For this review, take the finished solid that the model builds, in its own axes (mm). Face numbers are marked on the shaded views. A direction names the side the tool comes from. Round coordinates to 2 decimals unless told otherwise and drop trailing zeros. Loops run counter-clockwise (first coordinate to the right, second up) from the corner with the lowest first, then second, coordinate; pieces in that order, holes last. Notation, with made-up numbers: M 29.25,-28 L 83.25,-28 A14 cw 83.25,-13 Z; hole C 7,-20 d1. An arc over 180 degrees is marked long. One line per question, with ' | ' between items. Start each with the question number.
1) For pin 1 Ø1 at (y, z) = (1, 0) entering from -X; pin 2 Ø1.5 at (y, z) = (1, -8) entering from -X; pin 3 Ø1.5 at (x, y) = (-2, -2) entering from -Z, all flat-tipped, find the tip position at first contact; note any pin that passes through.
2) For the marked faces 1 and 2, list the 3-axis set-ups (+Z, -Z, +X, -X, +Y, -Y) from which the entire face can be reached by the end or side of a thin tool; tool diameter is ignored.
3) We need section A-A (y = 0). Give the boundary of the cut face in (x, z), and give its area (3 significant figures).
4) We need section B-B (z = 7.75). Give the boundary of the cut face in (x, y), and give its area (3 significant figures).
5) For probe 1 along X at (y, z) = (-0.1, 3.25); probe 2 along Z at (x, y) = (-0.9, 0.1); probe 3 along Z at (x, y) = (-2.15, 1.65), list the stretches that pass through material, from the lowest coordinate up. Write a range as from..to.
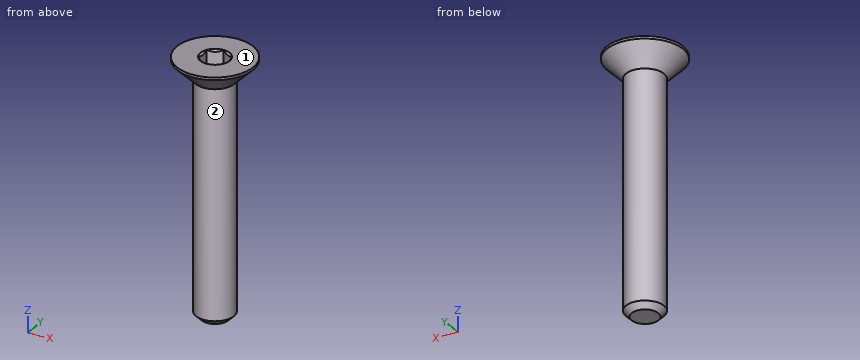
```python
from build123d import *

# Parameters (mm, degrees)
SKETCH3_W          = 20
SKETCH3_H          = 1.5
CHAMFER1_SIZE      = 0.45
CUT_EXTRUDE1_DEPTH = 1.19


with BuildPart() as part:
    # Sketch3 → Revolve1 (revolve)
    with BuildSketch(Plane(origin=(0, 0, 0), x_dir=(0, 0, -1), z_dir=(1, 0, 0))):
        with Locations((0, 0.75)):
            Rectangle(SKETCH3_W, SKETCH3_H)
    revolve(axis=Axis((0, 0, -10), (0, 0, 1)))

    # Chamfer1
    chamfer1_edges = [part.edges().sort_by_distance(p)[0] for p in [
        (0, -1.5, -10),
    ]]
    chamfer(chamfer1_edges, length=CHAMFER1_SIZE)

    # Sketch6 → Revolve2 (revolve)
    with BuildSketch(Plane(origin=(0, 0, 0), x_dir=(0, 0, -1), z_dir=(1, 0, 0))):
        Polygon((-10, 3), (-9.8, 3), (-8.3, 1.5), (-8.3, 0), (-10, 0), align=None)
    revolve(axis=Axis((0, 0, -10), (0, 0, 1)))

    # Sketch8 → Cut-Extrude1 (cut)
    with BuildSketch(Plane.XY.offset(10)):
        Polygon((0, 1.154700538), (-1, 0.577350269), (-1, -0.577350269), (0, -1.154700538), (1, -0.577350269), (1, 0.577350269), align=None)
    extrude(amount=-CUT_EXTRUDE1_DEPTH, mode=Mode.SUBTRACT)

    # Cut-Extrude2 cone 1 section (through the dimple's axis) → Cut-Extrude2 (revolve, cut)
    with BuildSketch(Plane(origin=(0, 0, 10), x_dir=(0, -1, 0), z_dir=(1, 0, 0))):
        Polygon((0, 0), (1.154700538, 0), (0, 1.154700538), align=None)
    revolve(axis=Axis((0, 0, 10), (0, 0, -1)), mode=Mode.SUBTRACT)


solid = part.part
```
Answers below:
1) pin 1: x = -1.41 | pin 2: x = -1.48 | pin 3: z = 8.88
2) face 1: +Z, +X, -X, +Y, -Y | face 2: -Z
3) outline: M -3,9.8 L -1.5,8.3 L -1.5,-9.55 L -1.05,-10 L 1.05,-10 L 1.5,-9.55 L 1.5,8.3 L 3,9.8 L 3,10 L 1.15,10 L 1,9.85 L 1,8.81 L -1,8.81 L -1,9.85 L -1.15,10 L -3,10 Z | area: 60.2 mm^2
4) outline: C 0,0 d3 | area: 7.07 mm^2
5) probe 1: -1.5..1.5 | probe 2: -10..8.81 | probe 3: 9.51..10
